Can you work these out from the model? Positions are in its coordinate system, mm. Face numbers are marked on the shaded views. A direction names the side the tool comes from. Give positions to 0.01 mm unless a question says otherwise; leave off trailing zeros. Write each loop counter-clockwise with the first axis right and the second up, starting at its lowest first coordinate (ties: lowest second). Pieces come first, ordered by that corner, then holes. Notation, with made-up numbers: M 10.5,-26.75 L 19.5,-26.75 A20 ccw 19.5,2.25 Z; hole C 58,17 d5. An arc over 180 degrees is marked long. Answer as CSV lines item,"result". Start each with the question number.
```python
from build123d import *

# Parameters (mm, degrees)
SKETCH1_W           = 30
SKETCH1_H           = 30
SKETCH1_R           = 7.5
SKETCH1_R_2         = 1.525
BOSS_EXTRUDE1_DEPTH = 2
SKETCH3_W           = 2
SKETCH3_H           = 10
BOSS_EXTRUDE2_DEPTH = 10
SKETCH4_W           = 12
SKETCH4_H           = 10
SKETCH4_R           = 2.025
BOSS_EXTRUDE3_DEPTH = 2
SKETCH5_W           = 4
SKETCH5_H           = 10
CUT_EXTRUDE1_DEPTH  = 32.527765541
FILLET1_R           = 2
FILLET2_R           = 1
FILLET3_R           = 1


with BuildPart() as part:
    # Sketch1 → Boss-Extrude1 (new body)
    with BuildSketch(Plane(origin=(0, 0, 0), x_dir=(1, 0, 0), z_dir=(0, 1, 0))):
        Rectangle(SKETCH1_W, SKETCH1_H)
        with Locations(Location((0, 0, 0), (0, 0, 270))):
            Circle(SKETCH1_R, mode=Mode.SUBTRACT)
        with Locations(Location((-7.778174593, 7.778174593, 0), (0, 0, 270))):
            Circle(SKETCH1_R_2, mode=Mode.SUBTRACT)
        with Locations(Location((7.778174593, 7.778174593, 0), (0, 0, 270))):
            Circle(SKETCH1_R_2, mode=Mode.SUBTRACT)
        with Locations(Location((-7.778174593, -7.778174593, 0), (0, 0, 270))):
            Circle(SKETCH1_R_2, mode=Mode.SUBTRACT)
        with Locations(Location((7.778174593, -7.778174593, 0), (0, 0, 270))):
            Circle(SKETCH1_R_2, mode=Mode.SUBTRACT)
    extrude(amount=BOSS_EXTRUDE1_DEPTH)

    # Sketch3 → Boss-Extrude2 (add)
    with BuildSketch(Plane.XZ):
        with Locations((-14, 10)):
            Rectangle(SKETCH3_W, SKETCH3_H)
        with Locations((14, 10)):
            Rectangle(SKETCH3_W, SKETCH3_H)
        with Locations((14, -10)):
            Rectangle(SKETCH3_W, SKETCH3_H)
        with Locations((-14, -10)):
            Rectangle(SKETCH3_W, SKETCH3_H)
    extrude(amount=BOSS_EXTRUDE2_DEPTH)

    # Sketch4 → Boss-Extrude3 (add)
    # profile 1 of 4: a face of its own
    with BuildSketch(Plane.XZ.offset(10)):
        with Locations((-19, 10)):
            Rectangle(SKETCH4_W, SKETCH4_H)
        with Locations(Location((-20, 10, 0), (0, 0, 270))):
            Circle(SKETCH4_R, mode=Mode.SUBTRACT)
    # profile 2 of 4: a face of its own
    with BuildSketch(Plane.XZ.offset(10)):
        with Locations((19, 10)):
            Rectangle(SKETCH4_W, SKETCH4_H)
        with Locations(Location((20, 10, 0), (0, 0, 90))):
            Circle(SKETCH4_R, mode=Mode.SUBTRACT)
    # profile 3 of 4: a face of its own
    with BuildSketch(Plane.XZ.offset(10)):
        with Locations((19, -10)):
            Rectangle(SKETCH4_W, SKETCH4_H)
        with Locations(Location((20, -10, 0), (0, 0, 270))):
            Circle(SKETCH4_R, mode=Mode.SUBTRACT)
    # profile 4 of 4: a face of its own
    with BuildSketch(Plane.XZ.offset(10)):
        with Locations((-19, -10)):
            Rectangle(SKETCH4_W, SKETCH4_H)
        with Locations(Location((-20, -10, 0), (0, 0, 90))):
            Circle(SKETCH4_R, mode=Mode.SUBTRACT)
    extrude(amount=BOSS_EXTRUDE3_DEPTH)

    # Sketch5 → Cut-Extrude1 (cut, through all)
    with BuildSketch(Plane.XZ):
        with Locations((-13, 0)):
            Rectangle(SKETCH5_W, SKETCH5_H)
        with Locations((13, 0)):
            Rectangle(SKETCH5_W, SKETCH5_H)
    extrude(amount=-CUT_EXTRUDE1_DEPTH, mode=Mode.SUBTRACT)

    # Fillet1
    fillet1_edges = [part.edges().sort_by_distance(p)[0] for p in [
        (13, -12, -10),
        (-13, -12, -10),
        (-15, 2, -10),
        (-15, 2, 10),
        (15, 2, -10),
        (15, 2, 10),
        (-13, -12, 10),
        (13, -12, 10),
    ]]
    fillet(fillet1_edges, radius=FILLET1_R)

    # Fillet2
    fillet2_edges = [part.edges().sort_by_distance(p)[0] for p in [
        (-13, 0, 10),
        (-15, -10, 10),
        (13, 0, 10),
        (15, -10, 10),
        (13, 0, -10),
        (15, -10, -10),
        (-13, 0, -10),
        (-15, -10, -10),
    ]]
    fillet(fillet2_edges, radius=FILLET2_R)

    # Fillet3
    fillet3_edges = [part.edges().sort_by_distance(p)[0] for p in [
        (-11, 1, -5),
        (11, 1, -5),
        (11, 1, 5),
        (-11, 1, 5),
    ]]
    fillet(fillet3_edges, radius=FILLET3_R)


solid = part.part
```
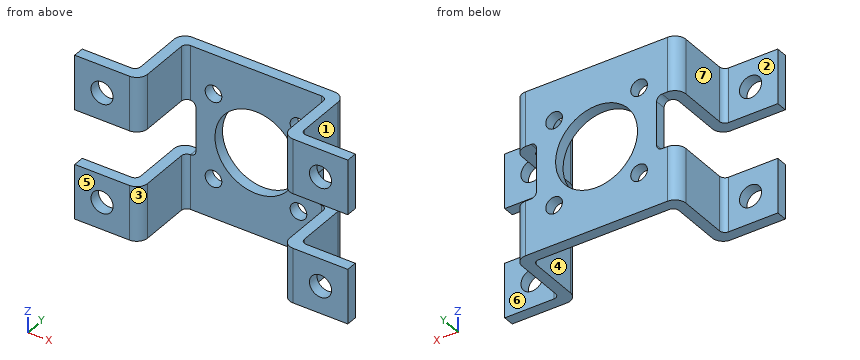
1) Thinking about a two-plate mould opening in X: for the marked faces 1, 2 and 3, which applies, released by +X, released by -X, zero draft, split by the parting line, or undercut?
2) I want a section at D-D, the plane z = -10. Please give me the cut outline in (x, y) (3 decimals).
3) I need wall thicknesses on L1, parallel to X at y = -7, z = 10; L2, parallel to X at y = -10.8, z = 10 (3 decimals); L3, parallel to X at y = -10.6, z = -10 (3 decimals). Which ranges of each line are inside material? Lowest first, please. Write a range as from..to.
4) I want a section at C-C, the plane z = 0. Please give me the cut outline in (x, y).
5) I want a section at B-B, the plane x = 16.5. Please give me the cut outline in (y, z), then the cut area to 3 significant figures.
6) On a 3-axis mill with a long thin cutter (end or side, diameter ignored), from which of +Z, -Z, +X, -X, +Y, -Y can I reach the whole of each face in a straight line? I mean the marked faces 4, 5, 6 and 7. Say none if no direction works.
7) I want a section at A-A, the plane y = -2.25. Please give me the cut outline in (x, z), then the cut area to 3 significant figures.
8) I'm going to push flat-ended pins straight in: P1, Ø4.5, axis at x = 19.5, z = -9, coming from the +Y side; P2, Ø2.5, axis at y = -5.5, z = 8, coming from the +X side; P3, Ø2.5, axis at x = 7.78, z = -7.78, coming from the +Y side; P4, Ø2.5, axis at y = -3, z = 8.5, coming from the -X side. Where does each tip first touch, or does it pass through?
Values found:
1,face 1,"released by +X"
1,face 2,"zero draft"
1,face 3,"undercut"
2,outline,"M -25,-12 L -22.025,-12 L -22.025,-10 L -25,-10 Z; M -17.975,-12 L -15,-12 A2 ccw -13,-10 L -13,-1 A1 cw -12,0 L 12,0 A1 cw 13,-1 L 13,-10 A2 ccw 15,-12 L 17.975,-12 L 17.975,-10 L 16,-10 A1 cw 15,-9 L 15,0 A2 ccw 13,2 L -13,2 A2 ccw -15,0 L -15,-9 A1 cw -16,-10 L -17.975,-10 Z; M 22.025,-12 L 25,-12 L 25,-10 L 22.025,-10 Z"
3,L1,"x = -15..-13, 13..15"
3,L2,"x = -25..-22.025, -17.975..-13.167, 13.167..17.975, 22.025..25"
3,L3,"x = -25..-22.025, -17.975..-13.092, 13.092..17.975, 22.025..25"
4,outline,"M -11,0 L -7.5,0 L -7.5,2 L -11,2 Z; M 7.5,0 L 11,0 L 11,2 L 7.5,2 Z"
5,outline,"M -12,-15 L -10,-15 L -10,-5 L -12,-5 Z; M -12,5 L -10,5 L -10,15 L -12,15 Z"
5,area,"40.0 mm²"
6,face 4,"+Z, -Z, -Y"
6,face 5,"+Z, -Z, +X, -X, -Y"
6,face 6,"+Z, -Z, +X, +Y"
6,face 7,"+Z, -Z, -X, +Y"
7,outline,"M -15,-15 L -13,-15 L -13,-5 L -15,-5 Z; M -15,5 L -13,5 L -13,15 L -15,15 Z; M 13,-15 L 15,-15 L 15,-5 L 13,-5 Z; M 13,5 L 15,5 L 15,15 L 13,15 Z"
7,area,"80.0 mm²"
8,P1,"stops at y = -10"
8,P2,"stops at x = 15"
8,P3,"passes through"
8,P4,"stops at x = -15"
